Here's how the part is built. I have some questions about the finished solid (model axes, mm). Face numbers are marked on the shaded views. Round coordinates to 2 decimals unless told otherwise and drop trailing zeros. Loops run counter-clockwise (first coordinate to the right, second up) from the corner with the lowest first, then second, coordinate; pieces in that order, holes last. Notation, with made-up numbers: M -10.5,9 L 33.5,9 A14 ccw 33.5,27 Z; hole C -38,-37 d8. An arc over 180 degrees is marked long. Answer as a JSON object with one key per item and string values.
from build123d import *

# Parameters (mm, degrees)
BOSS_EXTRUDE2_DEPTH = 5.4
SKETCH24_R          = 50
CUT_EXTRUDE1_DEPTH  = 342.837952203
SKETCH26_R          = 1.6
CUT_EXTRUDE2_DEPTH  = 8.2
SKETCH27_R          = 1.6
CUT_EXTRUDE3_DEPTH  = 8.2
SKETCH28_R          = 1.6
CUT_EXTRUDE4_DEPTH  = 8.2
SKETCH29_R          = 1.6
CUT_EXTRUDE5_DEPTH  = 8.2
SKETCH30_R          = 1.6
CUT_EXTRUDE6_DEPTH  = 8.2
SKETCH31_R          = 1.6
CUT_EXTRUDE7_DEPTH  = 8.2
SKETCH32_R          = 50
BOSS_EXTRUDE3_DEPTH = 10
CUT_EXTRUDE10_DEPTH = 8


with BuildPart() as part:
    # Sketch1 → Boss-Extrude2 (new body)
    with BuildSketch(Plane(origin=(0, 0, 0), x_dir=(1, 0, 0), z_dir=(0, 1, 0))):
        with BuildLine():
            Line((-213.563400388, 37.399198664), (-226.012295427, 37.399198664))
            Line((-226.012295427, 37.399198664), (-238.461190465, 37.399198664))
            Line((-238.461190465, 37.399198664), (-261.523434509, -2.545779757))
            Line((-261.523434509, -2.545779757), (-255.29898699, -13.326839109))
            Line((-255.29898699, -13.326839109), (-249.074539471, -24.107898462))
            ThreePointArc((-249.074539471, -24.107898462), (-185.740063438, -103.806428821), (-148.38634952, -198.50495918))
            Line((-148.38634952, -198.50495918), (-142.161902, -209.286018532))
            Line((-142.161902, -209.286018532), (-135.937454481, -220.067077885))
            Line((-135.937454481, -220.067077885), (-89.812966393, -220.067077885))
            Line((-89.812966393, -220.067077885), (-83.588518873, -209.286018532))
            Line((-83.588518873, -209.286018532), (-77.364071354, -198.50495918))
            ThreePointArc((-77.364071354, -198.50495918), (-40.010357435, -103.806428821), (23.324118597, -24.107898462))
            Line((23.324118597, -24.107898462), (29.548566116, -13.326839109))
            Line((29.548566116, -13.326839109), (35.773013636, -2.545779757))
            Line((35.773013636, -2.545779757), (12.710769592, 37.399198664))
            Line((12.710769592, 37.399198664), (0.261874553, 37.399198664))
            Line((0.261874553, 37.399198664), (-12.187020486, 37.399198664))
            ThreePointArc((-12.187020486, 37.399198664), (-112.875210437, 22.399198664), (-213.563400388, 37.399198664))
        make_face()
    extrude(amount=BOSS_EXTRUDE2_DEPTH)

    # Sketch24 → Cut-Extrude1 (cut, through all)
    with BuildSketch(Plane(origin=(0, 5.4, 0), x_dir=(1, 0, 0), z_dir=(0, 1, 0))):
        with Locations(Location((-112.875210437, -61.737886326, 0), (0, 0, 270))):
            Circle(SKETCH24_R)
    extrude(amount=-CUT_EXTRUDE1_DEPTH, mode=Mode.SUBTRACT)

    # Sketch26 → Cut-Extrude2 (cut)
    with BuildSketch(Plane(origin=(-197.244930853, 0, 113.879413924), x_dir=(0.5000000000000135, 0, 0.8660254037844309), z_dir=(-0.8660254037844309, 0, 0.5000000000000135))):
        with Locations((106.666057706, 2.5)):
            Circle(SKETCH26_R)
        with Locations((113.666057706, 2.5)):
            Circle(SKETCH26_R)
    extrude(amount=-CUT_EXTRUDE2_DEPTH, mode=Mode.SUBTRACT)

    # Sketch27 → Cut-Extrude3 (cut)
    with BuildSketch(Plane(origin=(-197.244930853, 0, 113.879413924), x_dir=(0.5000000000000427, 0, 0.8660254037844141), z_dir=(-0.8660254037844141, 0, 0.5000000000000427))):
        with Locations((-119.608112274, 2.5)):
            Circle(SKETCH27_R)
        with Locations((-112.608112274, 2.5)):
            Circle(SKETCH27_R)
    extrude(amount=-CUT_EXTRUDE3_DEPTH, mode=Mode.SUBTRACT)

    # Sketch28 → Cut-Extrude4 (cut)
    with BuildSketch(Plane(origin=(0, 0, -37.399198664), x_dir=(-1, 0, 0), z_dir=(0, 0, -1))):
        with Locations((222.512295427, 2.5)):
            Circle(SKETCH28_R)
        with Locations((229.512295427, 2.5)):
            Circle(SKETCH28_R)
    extrude(amount=-CUT_EXTRUDE4_DEPTH, mode=Mode.SUBTRACT)

    # Sketch29 → Cut-Extrude5 (cut)
    with BuildSketch(Plane(origin=(0, 0, -37.399198664), x_dir=(-1, 0, 0), z_dir=(0, 0, -1))):
        with Locations((-3.761874553, 2.5)):
            Circle(SKETCH29_R)
        with Locations((3.238125447, 2.5)):
            Circle(SKETCH29_R)
    extrude(amount=-CUT_EXTRUDE5_DEPTH, mode=Mode.SUBTRACT)

    # Sketch30 → Cut-Extrude6 (cut)
    with BuildSketch(Plane(origin=(27.932115198, 0, 16.126614228), x_dir=(0.5000000000001847, 0, -0.8660254037843321), z_dir=(0.866025403784332, 0, 0.5000000000001846))):
        with Locations((-0.267098163, 2.5)):
            Circle(SKETCH30_R)
        with Locations((6.732901837, 2.5)):
            Circle(SKETCH30_R)
    extrude(amount=-CUT_EXTRUDE6_DEPTH, mode=Mode.SUBTRACT)

    # Sketch31 → Cut-Extrude7 (cut)
    with BuildSketch(Plane(origin=(27.932115198, 0, 16.126614228), x_dir=(0.5000000000000033, 0, -0.8660254037844368), z_dir=(0.8660254037844367, 0, 0.5000000000000032))):
        with Locations((-226.541268142, 2.5)):
            Circle(SKETCH31_R)
        with Locations((-219.541268142, 2.5)):
            Circle(SKETCH31_R)
    extrude(amount=-CUT_EXTRUDE7_DEPTH, mode=Mode.SUBTRACT)

    # Sketch32 → Boss-Extrude3 (add)
    with BuildSketch(Plane(origin=(0, 5.4, 0), x_dir=(1, 0, 0), z_dir=(0, 1, 0))):
        with BuildLine():
            Line((-226.012295427, 37.399198664), (-213.563400388, 37.399198664))
            ThreePointArc((-213.563400388, 37.399198664), (-112.875210437, 22.399198664), (-12.187020486, 37.399198664))
            Line((-12.187020486, 37.399198664), (0.261874553, 37.399198664))
            Line((0.261874553, 37.399198664), (12.710769592, 37.399198664))
            Line((12.710769592, 37.399198664), (35.773013636, -2.545779757))
            Line((35.773013636, -2.545779757), (29.548566116, -13.326839109))
            Line((29.548566116, -13.326839109), (23.324118597, -24.107898462))
            ThreePointArc((23.324118597, -24.107898462), (-40.010357435, -103.806428821), (-77.364071354, -198.50495918))
            Line((-77.364071354, -198.50495918), (-83.588518873, -209.286018532))
            Line((-83.588518873, -209.286018532), (-89.812966393, -220.067077885))
            Line((-89.812966393, -220.067077885), (-135.937454481, -220.067077885))
            Line((-135.937454481, -220.067077885), (-142.161902, -209.286018532))
            Line((-142.161902, -209.286018532), (-148.38634952, -198.50495918))
            ThreePointArc((-148.38634952, -198.50495918), (-185.740063438, -103.806428821), (-249.074539471, -24.107898462))
            Line((-249.074539471, -24.107898462), (-255.29898699, -13.32683911))
            Line((-255.29898699, -13.32683911), (-261.523434509, -2.545779757))
            Line((-261.523434509, -2.545779757), (-238.461190465, 37.399198664))
            Line((-238.461190465, 37.399198664), (-226.012295427, 37.399198664))
        make_face()
        with Locations(Location((-112.875210437, -61.737886326, 0), (0, 0, 270))):
            Circle(SKETCH32_R, mode=Mode.SUBTRACT)
    extrude(amount=BOSS_EXTRUDE3_DEPTH)

    # Sketch36 → Cut-Extrude10 (cut)
    with BuildSketch(Plane.XZ):
        Polygon((-126.824859873, 209.850554734), (-137.330315468, 191.654571888), (-164.323687679, 91.441678511), (-237.613913024, 17.958285754), (-248.119368619, -0.237697092), (-234.169719182, -24.399198664), (-213.158807994, -24.399198664), (-112.875210437, 2.330301956), (-12.59161288, -24.399198664), (8.419298308, -24.399198664), (22.368947745, -0.237697092), (11.863492151, 17.958285754), (-61.426733195, 91.441678511), (-88.420105406, 191.654571888), (-98.925561, 209.850554734), align=None)
    extrude(amount=-CUT_EXTRUDE10_DEPTH, mode=Mode.SUBTRACT)


solid = part.part
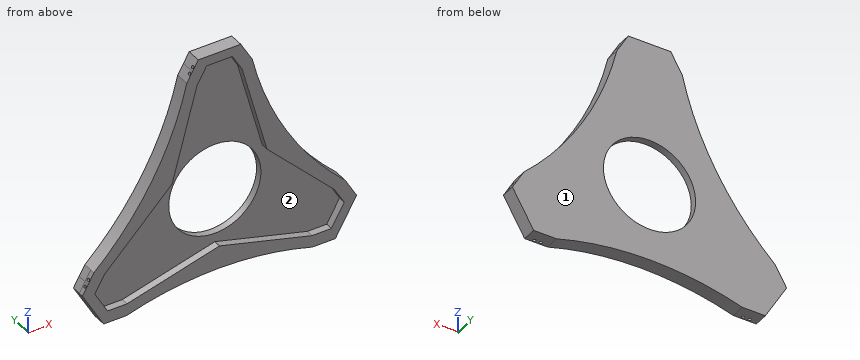
Item 1: If we mould it in two halves opening along Z, with no side actions, what happens to the marked faces 1 and 2? For each: pulls with the +Z half, pulls with the -Z half, needs draft (parallel to the pull), parting line crosses it, or undercut.
Resolved:
{"face 1": "needs draft", "face 2": "undercut"}
Item 2: Please list where these lines run through material, in increasing order: probe 1 along Z at (x, y) = (-112, 14.75); probe 2 along X at (y, z) = (14.25, 151.5); probe 3 along Y at (x, z) = (-41, -9.5). Write a range as from..to.
Resolved:
{"probe 1": "-22.4..11.75, 111.73..220.07", "probe 2": "-162.88..-62.87", "probe 3": "8..15.4"}
Item 3: I'm going to push flat-ended pins straight in: pin 1 Ø5 at (x, y) = (-222.51, 2.5) entering from +Z; pin 2 Ø2.5 at (x, y) = (-229.51, 2.5) entering from -Z; pin 3 Ø6.5 at (x, y) = (-111.5, 4) entering from -Z; pin 4 Ø1 at (x, z) = (-148.5, 94) entering from +Y. Where does each tip first touch, or does it pass through?
Resolved:
{"pin 1": "z = 54.8", "pin 2": "z = -29.2", "pin 3": "z = -22.43", "pin 4": "through"}
Item 4: I want a section at A-A, the plane z = -16. Please give me the cut outline in (x, y).
Resolved:
{"outline": "M -250.82,0 L -239.02,0 L -239.02,8 L -181.65,8 L -181.65,0 L -44.1,0 L -44.1,8 L 13.27,8 L 13.27,0 L 25.07,0 L 25.07,15.4 L -250.82,15.4 Z"}
